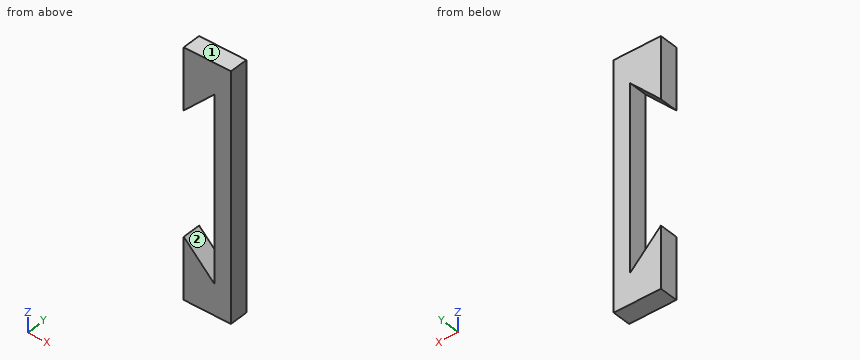
```python
from build123d import *

# Parameters (mm, degrees)
CROQUIS1_R                 = 11
CROQUIS1_R_2               = 2
CROQUIS1_R_3               = 1.937672591
CROQUIS1_W                 = 30
CROQUIS1_H                 = 3
SALIENTE_EXTRUIR1_DEPTH    = 3
CROQUIS2_R                 = 13
CROQUIS2_R_2               = 11
SALIENTE_EXTRUIR2_DEPTH    = 4
CROQUIS3_R                 = 13
CROQUIS3_R_2               = 9
SALIENTE_EXTRUIR3_DEPTH    = 2
CHAFL_N1_SIZE              = 2
CHAFL_N2_SIZE              = 10
CORTAR_EXTRUIR1_DEPTH      = 10
CORTAR_EXTRUIR1_DEPTH_BACK = 10
CROQUIS4_W                 = 138.754626828
CROQUIS4_H                 = 77.213714618


with BuildPart() as part:
    # Croquis1 → Saliente-Extruir1 (new body)
    with BuildSketch(Plane(origin=(0, 0, 0), x_dir=(1, 0, 0), z_dir=(0, 1, 0))):
        Polygon((-67.5, 10), (-62.5, 15), (-62.5, -15), (-67.5, -10), (-67.5, -20), (67.5, -20), (67.5, 20), (-67.5, 20), align=None)
        with Locations(Location((46.713951104, 0, 0), (0, 0, 270))):
            Circle(CROQUIS1_R, mode=Mode.SUBTRACT)
        with Locations(Location((-52.5, 0, 0), (0, 0, 270))):
            Circle(CROQUIS1_R_2, mode=Mode.SUBTRACT)
        with Locations(Location((27.185770037, 0, 0), (0, 0, 270))):
            Circle(CROQUIS1_R_3, mode=Mode.SUBTRACT)
        with Locations(Location((12.185770037, 0, 0), (0, 0, 270))):
            Circle(CROQUIS1_R_2, mode=Mode.SUBTRACT)
        with Locations((-27.5, 11)):
            Rectangle(CROQUIS1_W, CROQUIS1_H, mode=Mode.SUBTRACT)
        with Locations((-27.5, -11)):
            Rectangle(CROQUIS1_W, CROQUIS1_H, mode=Mode.SUBTRACT)
    extrude(amount=SALIENTE_EXTRUIR1_DEPTH)

    # Croquis2 → Saliente-Extruir2 (add)
    with BuildSketch(Plane(origin=(0, 3, 0), x_dir=(1, 0, 0), z_dir=(0, 1, 0))):
        with Locations(Location((46.713951104, 0, 0), (0, 0, 90))):
            Circle(CROQUIS2_R)
        with Locations(Location((46.713951104, 0, 0), (0, 0, 270))):
            Circle(CROQUIS2_R_2, mode=Mode.SUBTRACT)
    extrude(amount=SALIENTE_EXTRUIR2_DEPTH)

    # Croquis3 → Saliente-Extruir3 (add)
    with BuildSketch(Plane(origin=(0, 7, 0), x_dir=(1, 0, 0), z_dir=(0, 1, 0))):
        with Locations(Location((46.713951104, 0, 0), (0, 0, 90))):
            Circle(CROQUIS3_R)
        with Locations(Location((46.713951104, 0, 0), (0, 0, 270))):
            Circle(CROQUIS3_R_2, mode=Mode.SUBTRACT)
    extrude(amount=SALIENTE_EXTRUIR3_DEPTH)

    # Chafl_n1
    chafl_n1_edges = [part.edges().sort_by_distance(p)[0] for p in [
        (46.713951104, 9, 13),
    ]]
    chamfer(chafl_n1_edges, length=CHAFL_N1_SIZE)

    # Chafl_n2
    chafl_n2_edges = [part.edges().sort_by_distance(p)[0] for p in [
        (67.5, 1.5, 20),
        (67.5, 1.5, -20),
    ]]
    chamfer(chafl_n2_edges, length=CHAFL_N2_SIZE)

    # Croquis4 → Cortar-Extruir1 (cut, two sides: drawn at the far end of the back side and taken through both)
    with BuildSketch(Plane(origin=(0, 3, 0), x_dir=(1, 0, 0), z_dir=(0, 1, 0)).offset(-CORTAR_EXTRUIR1_DEPTH_BACK)):
        with Locations((9.561847341, -1.869233315)):
            Rectangle(CROQUIS4_W, CROQUIS4_H)
    extrude(amount=CORTAR_EXTRUIR1_DEPTH + CORTAR_EXTRUIR1_DEPTH_BACK, mode=Mode.SUBTRACT)


solid = part.part
```
Part model, mm, in its own coordinate system. Face numbers are marked on the shaded views. Round coordinates to 2 decimals unless told otherwise and drop trailing zeros. Order: outer loops, then holes, each group sorted by start corner. A loop starts at its lowest first (then second) coordinate and runs counter-clockwise, first axis right, second up. Notation, with made-up numbers: M -1,-2.5 L 50,-2.5 A17 cw 50,7.5 Z; hole C 4.5,-5.75 d8. An arc over 180 degrees is marked long. Put each result on its own line as item: value. Start each with the question number.
1. Two-plate mould, pull along X, no slides. Class the marked faces 1 and 2: +X half, -X half, draft (parallel to the pull), parting line (faces both ways), or undercut.
2. Slice it at D-D on z = 4. List the corners of the cut face in (x, y), then the cut area to 3 significant figures.
3. Drill centre lines: probe 1 along X at (y, z) = (0.9, 3); probe 2 along Z at (x, y) = (-65.75, 0.75); probe 3 along Z at (x, y) = (-63.5, 2.55). Where is each one in solid material? Low to high. Write a range as [from, to].
4. Slice it at B-B on z = 12. List the corners of the cut face in (x, y), then the cut area to 3 significant figures.
5. Slice it at A-A on x = -63.5. List the corners of the cut face in (y, z).
6. Slice it at C-C on y = 0.7. List the corners of the cut face in (x, z).
Findings:
1. face 1: draft
1. face 2: undercut
2. outline: M -62.5,0 L -59.82,0 L -59.82,3 L -62.5,3 Z
2. area: 8.05 mm2
3. probe 1: [-62.5, -59.82]
3. probe 2: [-20, -11.75], [11.75, 20]
3. probe 3: [-20, -14], [14, 20]
4. outline: M -67.5,0 L -65.5,0 L -65.5,3 L -67.5,3 Z; M -62.5,0 L -59.82,0 L -59.82,3 L -62.5,3 Z
4. area: 14.1 mm2
5. outline: M 0,-20 L 3,-20 L 3,-14 L 0,-14 Z; M 0,14 L 3,14 L 3,20 L 0,20 Z
6. outline: M -67.5,-20 L -59.82,-20 L -59.82,20 L -67.5,20 L -67.5,10 L -62.5,15 L -62.5,-15 L -67.5,-10 Z
